Design review of the part built by this model. Coordinates are the model's own, in mm. Face numbers are marked on the shaded views. Round coordinates to 2 decimals unless told otherwise and drop trailing zeros. Order: outer loops, then holes, each group sorted by start corner. A loop starts at its lowest first (then second) coordinate and runs counter-clockwise, first axis right, second up. Notation, with made-up numbers: (53, 32) - (65, 32) arc R27 ccw to (65, 62) - close; hole circle Ø9 at (48.5, 19.5). An arc over 180 degrees is marked (long way). Use CSV: the item, a comma, the result in double quotes. Start each with the question number.
from build123d import *

# Parameters (mm, degrees)
F0_R     = 7.5
F1_DEPTH = 79
F2_T     = -2
F3_SIZE  = 1


with BuildPart() as f1:
    # F0 (on Top) → F1 (new body)
    with BuildSketch(Plane.XY):
        Circle(F0_R)
    extrude(amount=F1_DEPTH)

    # F2
    f2_openings = [f1.faces().sort_by_distance(p)[0] for p in [
        (0, 0, 79),
        (0, 0, 0),
    ]]
    offset(amount=F2_T, openings=f2_openings)

    # F3
    f3_edges = [f1.edges().sort_by_distance(p)[0] for p in [
        (-7.5, 0, 0),
        (-7.5, 0, 79),
    ]]
    chamfer(f3_edges, length=F3_SIZE)


solid = f1.part
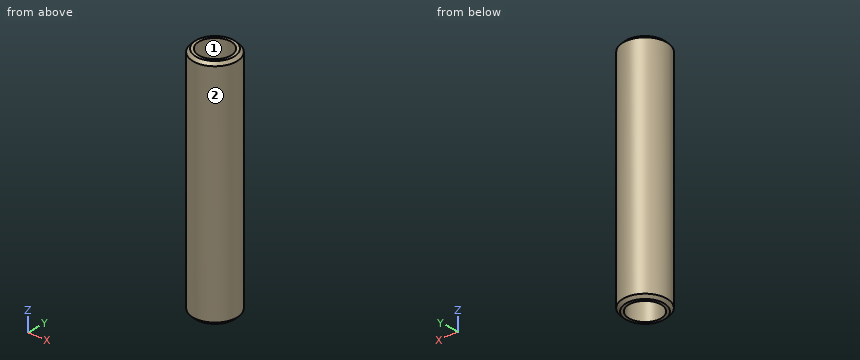
Q1. Take a section at A-A (x = 0). State the section outline as (y, z) points.
Q2. Take a section at C-C (z = 5). State the section outline as (x, y) points, plus the area to 3 significant figures.
Q3. Clearance check with flat-ended pins moving along their axes: pin 1 (1.5 mm diameter, centred on x = -5, y = -1, fed in from +Z); pin 2 (6.5 mm diameter, centred on x = 0, y = 0, fed in from -Z); pin 3 (8 mm diameter, centred on x = -5.5, z = 21.5, fed in from +Y). State where each tip first meets the part, or that it passes through.
Q4. For L1, parallel to Y at x = 0, z = 59; L2, parallel to Y at x = -1, z = 36.5, list the stretches that pass through material, from the lowest coordinate up. Write a range as [from, to].
Q5. The part is to be moulded in two halves that separate along Y. For the marked faces 1 and 2, say which applies: +Y half, -Y half, draft (parallel to the pull), parting line (faces both ways), or undercut.
Findings below:
1,outline,"(-7.5, 1) - (-6.5, 0) - (-5.5, 0) - (-5.5, 79) - (-6.5, 79) - (-7.5, 78) - close; (5.5, 0) - (6.5, 0) - (7.5, 1) - (7.5, 78) - (6.5, 79) - (5.5, 79) - close"
2,outline,"circle Ø15 at (0, 0); hole circle Ø11 at (0, 0)"
2,area,"81.7 mm^2"
3,pin 1,"stops at z = 79"
3,pin 2,"passes through"
3,pin 3,"stops at y = 7.35"
4,L1,"y = [-7.5, -5.5], [5.5, 7.5]"
4,L2,"y = [-7.43, -5.41], [5.41, 7.43]"
5,face 1,"undercut"
5,face 2,"parting line"
